Part model, mm, in its own coordinate system. A direction names the side the tool comes from. Give positions to 0.01 mm unless a question says otherwise; leave off trailing zeros. Write each loop counter-clockwise with the first axis right and the second up, starting at its lowest first coordinate (ties: lowest second). Pieces come first, ordered by that corner, then holes.
```python
from build123d import *

# Parameters (mm, degrees)
BOSS_EXTRUDE1_DEPTH = 50
SKETCH3_R           = 8.75
CUT_EXTRUDE1_DEPTH  = 50
SKETCH5_R           = 2.5
CUT_EXTRUDE3_DEPTH  = 10
SKETCH6_R           = 2.5
CUT_EXTRUDE4_DEPTH  = 10


with BuildPart() as part:
    # Sketch2 → Boss-Extrude1 (new body)
    with BuildSketch(Plane(origin=(0, 0, 0), x_dir=(1, 0, 0), z_dir=(0, 1, 0))):
        with BuildLine():
            Line((-54.874212294, -102.775031025), (47.605671551, -102.775031025))
            Line((47.605671551, -102.775031025), (59.453092269, -93.575105898))
            ThreePointArc((59.453092269, -93.575105898), (72.038989389, -72.419691965), (93.194403322, -59.833794845))
            Line((93.194403322, -59.833794845), (102.394328449, -47.986374127))
            Line((102.394328449, -47.986374127), (102.394328449, 56.694970167))
            Line((102.394328449, 56.694970167), (102.394328449, 102.013625873))
            Line((102.394328449, 102.013625873), (107.394328449, 102.013625873))
            Line((107.394328449, 102.013625873), (107.394328449, 122.013625873))
            Line((107.394328449, 122.013625873), (102.394328449, 122.013625873))
            Line((102.394328449, 122.013625873), (102.394328449, 109.513625873))
            Line((102.394328449, 109.513625873), (87.394328449, 104.513625873))
            Line((87.394328449, 104.513625873), (52.394328449, 104.513625873))
            Line((52.394328449, 104.513625873), (52.394328449, 69.513625873))
            Line((52.394328449, 69.513625873), (87.394328449, 69.513625873))
            Line((87.394328449, 69.513625873), (87.394328449, -42.846257379))
            Line((87.394328449, -42.846257379), (84.095735231, -47.094098648))
            ThreePointArc((84.095735231, -47.094098648), (61.432387672, -61.813090248), (46.713396072, -84.476437807))
            Line((46.713396072, -84.476437807), (42.465554802, -87.775031025))
            Line((42.465554802, -87.775031025), (-69.894328449, -87.775031025))
            Line((-69.894328449, -87.775031025), (-69.894328449, -52.775031025))
            Line((-69.894328449, -52.775031025), (-104.894328449, -52.775031025))
            Line((-104.894328449, -52.775031025), (-104.894328449, -87.775031025))
            Line((-104.894328449, -87.775031025), (-109.894328449, -102.775031025))
            Line((-109.894328449, -102.775031025), (-122.394328449, -102.775031025))
            Line((-122.394328449, -102.775031025), (-122.394328449, -107.775031025))
            Line((-122.394328449, -107.775031025), (-102.394328449, -107.775031025))
            Line((-102.394328449, -107.775031025), (-102.394328449, -102.775031025))
            Line((-102.394328449, -102.775031025), (-54.874212294, -102.775031025))
        make_face()
    extrude(amount=BOSS_EXTRUDE1_DEPTH)

    # Sketch3 → Cut-Extrude1 (cut)
    with BuildSketch(Plane(origin=(0, 50, 0), x_dir=(1, 0, 0), z_dir=(0, 1, 0))):
        with Locations((-87.394328449, -70.275031025)):
            Circle(SKETCH3_R)
        with Locations((69.894328449, 87.013625873)):
            Circle(SKETCH3_R)
    extrude(amount=-CUT_EXTRUDE1_DEPTH, mode=Mode.SUBTRACT)

    # Sketch5 → Cut-Extrude3 (cut)
    with BuildSketch(Plane(origin=(0, 0, 102.775031025), x_dir=(-1, 0, 0), z_dir=(0, 0, -1))):
        with Locations((116.144328449, 37.5)):
            Circle(SKETCH5_R)
        with Locations((116.144328449, 25)):
            Circle(SKETCH5_R)
        with Locations((116.144328449, 12.5)):
            Circle(SKETCH5_R)
    extrude(amount=-CUT_EXTRUDE3_DEPTH, mode=Mode.SUBTRACT)

    # Sketch6 → Cut-Extrude4 (cut)
    with BuildSketch(Plane.ZY.offset(-102.394328449)):
        with Locations((-115.763625873, 37.5)):
            Circle(SKETCH6_R)
        with Locations((-115.763625873, 25)):
            Circle(SKETCH6_R)
        with Locations((-115.763625873, 12.5)):
            Circle(SKETCH6_R)
    extrude(amount=-CUT_EXTRUDE4_DEPTH, mode=Mode.SUBTRACT)


solid = part.part
```
1) 3-axis set-ups, long thin cutter, end or side, ignore diameter. For faces 5 (the face through (102.394, 25, -119)), 6 (the face through (102.394, 25, -26)), 7 (the face through (87.394, 25, -14)): which of +Z, -Z, +X, -X, +Y, -Y reach the whole face in a straight line?
Answers follow:
face 5: -Z, -X, +Y, -Y
face 6: +Z, +X, +Y, -Y
face 7: -X, +Y, -Y
2) Saw through at C-C, the plane x = -5.5. Write the cut outline in (y, z), then the cut area to 3 significant figures.
Answers follow:
outline: (0, 87.78) - (50, 87.78) - (50, 102.78) - (0, 102.78) - close
area: 750 mm2
3) Saw through at D-D, the plane z = -8. Write the cut outline in (x, y), then the cut area to 3 significant figures.
Answers follow:
outline: (87.39, 0) - (102.39, 0) - (102.39, 50) - (87.39, 50) - close
area: 750 mm2
4) Saw through at A-A, the plane y = 4. Write the cut outline in (x, z).
Answers follow:
outline: (-122.39, 102.78) - (-109.89, 102.78) - (-104.89, 87.78) - (-104.89, 52.78) - (-69.89, 52.78) - (-69.89, 87.78) - (42.47, 87.78) - (46.71, 84.48) arc R65 ccw to (84.1, 47.09) - (87.39, 42.85) - (87.39, -69.51) - (52.39, -69.51) - (52.39, -104.51) - (87.39, -104.51) - (102.39, -109.51) - (102.39, -122.01) - (107.39, -122.01) - (107.39, -102.01) - (102.39, -102.01) - (102.39, 47.99) - (93.19, 59.83) arc R50 cw to (59.45, 93.58) - (47.61, 102.78) - (-102.39, 102.78) - (-102.39, 107.78) - (-122.39, 107.78) - close; hole circle Ø17.5 at (-87.39, 70.28); hole circle Ø17.5 at (69.89, -87.01)
5) Wall check: L1, parallel to Z at x = 105, y = 37; L2, parallel to X at y = 44, z = 73.5; L3, parallel to Z at x = -43, y = 10. Give the ranges that are in metal, low to high.
Answers follow:
L1: z = -122.01 to -118.21, -113.31 to -102.01
L2: x = -104.89 to -95.53, -79.26 to -69.89, 52.17 to 70.99
L3: z = 87.78 to 102.78
6) Pin check, flat tips, straight feed: pin 1 Ø1 at (x, y) = (35, 17) entering from +Z; pin 2 Ø12 at (y, z) = (15, -83) entering from -X; pin 3 Ø12 at (y, z) = (13, -14) entering from -X. Stop position of each tip, or through.
Answers follow:
pin 1: stops at z = 102.78
pin 2: stops at x = 52.39
pin 3: stops at x = 87.39
7) Two-plate mould, pull along Y, no slides. Class faces 1 (the face through (-102.394, 25, 105)), 2 (the face through (69, 0, 60)), 3 (the face through (-118.454, 11.542, 105.24)), 4 (the face through (104.86, 12.61, -118.26)): +Y half, -Y half, draft (parallel to the pull), parting line (faces both ways), or undercut.
Answers follow:
face 1: draft
face 2: -Y half
face 3: undercut
face 4: undercut
8) Saw through at B-B, the plane x = 67. Write the cut outline in (y, z).
Answers follow:
outline: (0, -104.51) - (50, -104.51) - (50, -95.27) - (0, -95.27) - close; (0, -78.76) - (50, -78.76) - (50, -69.51) - (0, -69.51) - close; (0, 56.85) - (50, 56.85) - (50, 78.31) - (0, 78.31) - close
